Could you check a few things on this model? Use its own coordinates, in mm. Round coordinates to 2 decimals unless told otherwise and drop trailing zeros. Loops run counter-clockwise (first coordinate to the right, second up) from the corner with the lowest first, then second, coordinate; pieces in that order, holes last. Notation, with made-up numbers: (42, 89.25) - (84, 89.25) arc R25 cw to (84, 124.25) - close; hole circle Ø8 at (-14.75, -37.5). An arc over 180 degrees is marked (long way). Answer as CSV lines item,"result". Start each with the question number.
1) Please list where these lines run through material, in increasing order: line 1 along Z through (x, y) = (-30.5, 1.7); line 2 along X through (y, z) = (0.3, 2); line 3 along Z through (x, y) = (-53.25, 2.1).
2) Suppose I cut it at A-A, the plane z = -16. Write out the boundary of the cut face in (x, y).
3) Suppose I cut it at C-C, the plane y = 1.55. Write out the boundary of the cut face in (x, z), then the cut area to 3 significant figures.
4) Suppose I cut it at B-B, the plane x = -37. Write out the boundary of the cut face in (y, z), then the cut area to 3 significant figures.
```python
from build123d import *

# Parameters (mm, degrees)
SKETCH1_R           = 1.1
SKETCH1_W           = 103
SKETCH1_H           = 90.5
BOSS_EXTRUDE1_DEPTH = 3


with BuildPart() as part:
    # Sketch1 → Boss-Extrude1 (new body)
    with BuildSketch(Plane(origin=(0, 0, 0), x_dir=(1, 0, 0), z_dir=(0, 1, 0))):
        with BuildLine():
            Line((-51.5, -50.25), (51.5, -50.25))
            ThreePointArc((51.5, -50.25), (55.035533906, -48.785533906), (56.5, -45.25))
            Line((56.5, -45.25), (56.5, 45.25))
            ThreePointArc((56.5, 45.25), (55.035533906, 48.785533906), (51.5, 50.25))
            Line((51.5, 50.25), (-51.5, 50.25))
            ThreePointArc((-51.5, 50.25), (-55.035533906, 48.785533906), (-56.5, 45.25))
            Line((-56.5, 45.25), (-56.5, -45.25))
            ThreePointArc((-56.5, -45.25), (-55.035533906, -48.785533906), (-51.5, -50.25))
        make_face()
        with Locations((-53.25, 47.25)):
            Circle(SKETCH1_R, mode=Mode.SUBTRACT)
        with Locations((53.25, 47.25)):
            Circle(SKETCH1_R, mode=Mode.SUBTRACT)
        with Locations((53.25, -47.25)):
            Circle(SKETCH1_R, mode=Mode.SUBTRACT)
        with Locations((-53.25, -47.25)):
            Circle(SKETCH1_R, mode=Mode.SUBTRACT)
        Rectangle(SKETCH1_W, SKETCH1_H, mode=Mode.SUBTRACT)
    extrude(amount=BOSS_EXTRUDE1_DEPTH)


solid = part.part
```
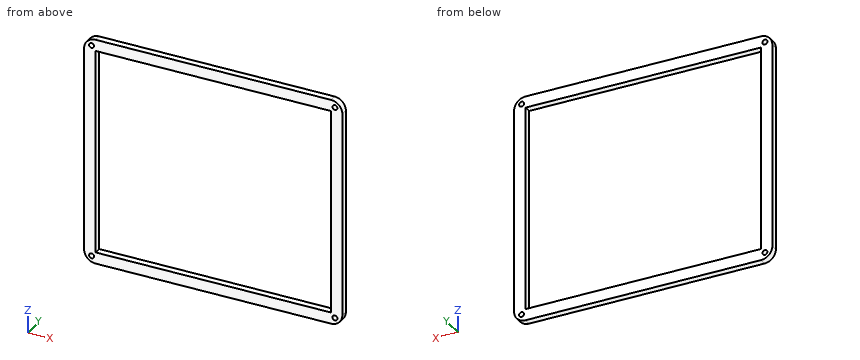
Filled sheet:
1,line 1,"-50.25 to -45.25, 45.25 to 50.25"
1,line 2,"-56.5 to -51.5, 51.5 to 56.5"
1,line 3,"-49.93 to -48.35, -46.15 to 46.15, 48.35 to 49.93"
2,outline,"(-56.5, 0) - (-51.5, 0) - (-51.5, 3) - (-56.5, 3) - close; (51.5, 0) - (56.5, 0) - (56.5, 3) - (51.5, 3) - close"
3,outline,"(-56.5, -45.25) arc R5 ccw to (-51.5, -50.25) - (51.5, -50.25) arc R5 ccw to (56.5, -45.25) - (56.5, 45.25) arc R5 ccw to (51.5, 50.25) - (-51.5, 50.25) arc R5 ccw to (-56.5, 45.25) - close; hole circle Ø2.2 at (-53.25, -47.25); hole circle Ø2.2 at (-53.25, 47.25); hole (-51.5, -45.25) - (51.5, -45.25) - (51.5, 45.25) - (-51.5, 45.25) - close; hole circle Ø2.2 at (53.25, -47.25); hole circle Ø2.2 at (53.25, 47.25)"
3,area,"2,000 mm²"
4,outline,"(0, -50.25) - (3, -50.25) - (3, -45.25) - (0, -45.25) - close; (0, 45.25) - (3, 45.25) - (3, 50.25) - (0, 50.25) - close"
4,area,"30.0 mm²"
